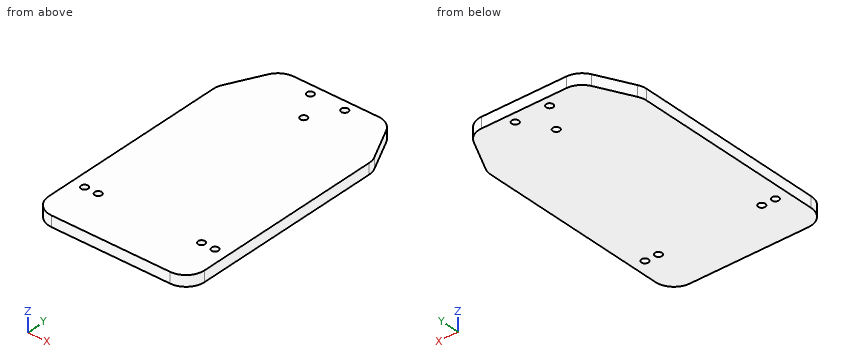
```python
from build123d import *

# Parameters (mm, degrees)
BOSS_EXTRUDE1_DEPTH = 6.35
SKETCH2_R           = 2.05
CUT_EXTRUDE1_DEPTH  = 6.35


with BuildPart() as part:
    # Sketch1 → Boss-Extrude1 (new body)
    with BuildSketch(Plane.XY):
        with BuildLine():
            Line((55, 144.8), (30, 144.8))
            ThreePointArc((30, 144.8), (24.216957767, 143.157158892), (20.161300899, 138.71934955))
            Line((20.161300899, 138.71934955), (10.161300899, 118.71934955))
            ThreePointArc((10.161300899, 118.71934955), (9.294261116, 116.327282126), (9, 113.8))
            Line((9, 113.8), (9, 0))
            ThreePointArc((9, 0), (12.221825407, -7.778174593), (20, -11))
            Line((20, -11), (90, -11))
            ThreePointArc((90, -11), (97.778174593, -7.778174593), (101, 0))
            Line((101, 0), (101, 113.8))
            ThreePointArc((101, 113.8), (100.705738884, 116.327282126), (99.838699101, 118.71934955))
            Line((99.838699101, 118.71934955), (89.838699101, 138.71934955))
            ThreePointArc((89.838699101, 138.71934955), (85.783042233, 143.157158892), (80, 144.8))
            Line((80, 144.8), (55, 144.8))
        make_face()
    extrude(amount=BOSS_EXTRUDE1_DEPTH)

    # Sketch2 → Cut-Extrude1 (cut)
    with BuildSketch(Plane.XY.offset(6.35)):
        with Locations((16.5, 16)):
            Circle(SKETCH2_R)
        with Locations((24.5, 16)):
            Circle(SKETCH2_R)
        with Locations((85.5, 16)):
            Circle(SKETCH2_R)
        with Locations((93.5, 16)):
            Circle(SKETCH2_R)
        with Locations((44.84, 138.898469816)):
            Circle(SKETCH2_R)
        with Locations((55, 122.428157316)):
            Circle(SKETCH2_R)
        with Locations((65.16, 138.898469816)):
            Circle(SKETCH2_R)
    extrude(amount=-CUT_EXTRUDE1_DEPTH, mode=Mode.SUBTRACT)


solid = part.part
```
Geometry check sheet. Reference: the model listing, model coordinates, mm. Coordinates: 2 decimals unless noted, no trailing zeros. Order: outer loops, then holes, each group sorted by start corner. A loop starts at its lowest first (then second) coordinate and runs counter-clockwise, first axis right, second up.
Item 1: Scan lines: line 1 along Y through (x, z) = (65.16, 3.5); line 2 along X through (y, z) = (15, 4.75); line 3 along Y through (x, z) = (55, 2.5). Record each from-to range of solid material in increasing order.
Item 2: Section check B-B (y = 16). Enter the section's corners in (x, z), plus the area to 3 significant figures.
Item 3: Depth check by flat-ended pin: pin 1 (3.5 mm diameter, centred on x = 55, y = 122.43, fed in from -Z). Enter the tip coordinate at first touch or a pass-through.
Item 4: Section check C-C (z = 3.25). Enter the section's corners in (x, y), plus the area to 3 significant figures.
Item 5: Section check D-D (x = 24.5). Enter the section's corners in (y, z), plus the area to 3 significant figures.
Item 6: Section check A-A (x = 55). Enter the section's corners in (y, z).
Check sheet entries:
1. line 1: y = -11 to 136.85, 140.95 to 144.8
1. line 2: x = 9 to 14.71, 18.29 to 22.71, 26.29 to 83.71, 87.29 to 91.71, 95.29 to 101
1. line 3: y = -11 to 120.38, 124.48 to 144.8
2. outline: (9, 0) - (14.45, 0) - (14.45, 6.35) - (9, 6.35) - close; (18.55, 0) - (22.45, 0) - (22.45, 6.35) - (18.55, 6.35) - close; (26.55, 0) - (83.45, 0) - (83.45, 6.35) - (26.55, 6.35) - close; (87.55, 0) - (91.45, 0) - (91.45, 6.35) - (87.55, 6.35) - close; (95.55, 0) - (101, 0) - (101, 6.35) - (95.55, 6.35) - close
2. area: 480 mm2
3. pin 1: passes through
4. outline: (9, 0) arc R11 ccw to (20, -11) - (90, -11) arc R11 ccw to (101, 0) - (101, 113.8) arc R11 ccw to (99.84, 118.72) - (89.84, 138.72) arc R11 ccw to (80, 144.8) - (30, 144.8) arc R11 ccw to (20.16, 138.72) - (10.16, 118.72) arc R11 ccw to (9, 113.8) - close; hole circle Ø4.1 at (16.5, 16); hole circle Ø4.1 at (24.5, 16); hole circle Ø4.1 at (44.84, 138.9); hole circle Ø4.1 at (55, 122.43); hole circle Ø4.1 at (65.16, 138.9); hole circle Ø4.1 at (85.5, 16); hole circle Ø4.1 at (93.5, 16)
4. area: 13,800 mm2
5. outline: (-11, 0) - (13.95, 0) - (13.95, 6.35) - (-11, 6.35) - close; (18.05, 0) - (143.33, 0) - (143.33, 6.35) - (18.05, 6.35) - close
5. area: 954 mm2
6. outline: (-11, 0) - (120.38, 0) - (120.38, 6.35) - (-11, 6.35) - close; (124.48, 0) - (144.8, 0) - (144.8, 6.35) - (124.48, 6.35) - close
